Geometry: see drawing. Coordinates: mm, zero at the bounding-box minimum. A direction names the side the tool comes from. Coordinates: 2 decimals unless noted, no trailing zeros. Order: outer loops, then holes, each group sorted by start corner. A loop starts at its lowest first (then second) coordinate and runs counter-clockwise, first axis right, second up.
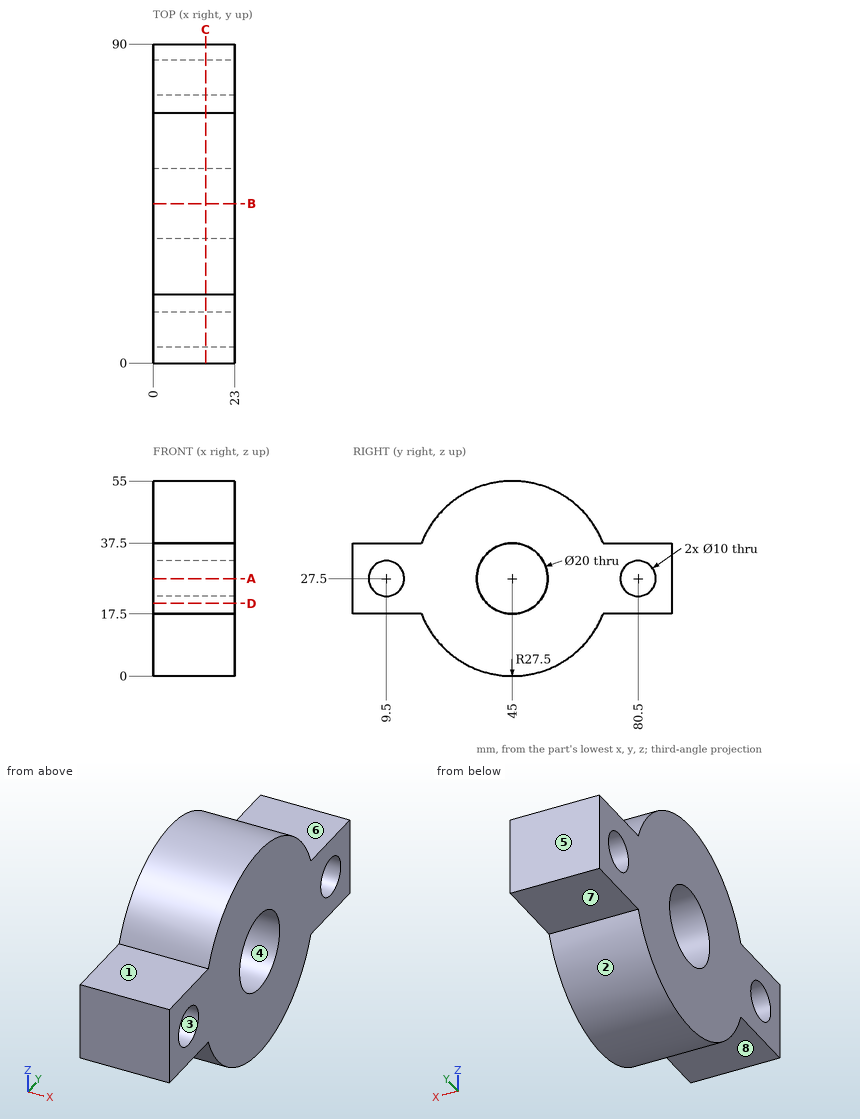
Q1. Section query B-B on y = 45. Output: boundary loops of the cut face in (x, z), plus the area to 3 significant figures.
Solutions:
outline: (0, 0) - (23, 0) - (23, 17.5) - (0, 17.5) - close; (0, 37.5) - (23, 37.5) - (23, 55) - (0, 55) - close
area: 805 mm2
Q2. Section query D-D on z = 20.5. Output: boundary loops of the cut face in (x, y), plus the area to 3 significant figures.
Solutions:
outline: (0, 0) - (23, 0) - (23, 37.86) - (0, 37.86) - close; (0, 52.14) - (23, 52.14) - (23, 90) - (0, 90) - close
area: 1,740 mm2
Q3. Material intervals for line 1 along Z through (x, y) = (11, 80.5); line 2 along Y through (x, z) = (17.5, 29); line 3 along Z through (x, y) = (3, 85), sorted ascending.
Solutions:
line 1: z = 17.5 to 22.5, 32.5 to 37.5
line 2: y = 0 to 4.73, 14.27 to 35.11, 54.89 to 75.73, 85.27 to 90
line 3: z = 17.5 to 25.32, 29.68 to 37.5
Q4. Pull-direction query (Z, two-part tool) for the marked faces 1, 2, 3 and 4; classes: pulls with the +Z half, pulls with the -Z half, needs draft (parallel to the pull), parting line crosses it, or undercut.
Solutions:
face 1: pulls with the +Z half
face 2: pulls with the -Z half
face 3: undercut
face 4: undercut
Q5. Set-up query: the marked faces 5, 6, 7 and 8. Return all of +Z, -Z, +X, -X, +Y, -Y with unobstructed straight access to the full face (end or side cutting, diameter ignored); none if empty.
Solutions:
face 5: +Z, -Z, +X, -X, +Y
face 6: +Z, +X, -X, +Y
face 7: -Z, +X, -X, +Y
face 8: -Z, +X, -X, -Y
Q6. Section query A-A on z = 27.5. Output: boundary loops of the cut face in (x, y), plus the area to 3 significant figures.
Solutions:
outline: (0, 0) - (23, 0) - (23, 4.5) - (0, 4.5) - close; (0, 14.5) - (23, 14.5) - (23, 35) - (0, 35) - close; (0, 55) - (23, 55) - (23, 75.5) - (0, 75.5) - close; (0, 85.5) - (23, 85.5) - (23, 90) - (0, 90) - close
area: 1,150 mm2
Q7. Section query C-C on x = 14.75. Output: boundary loops of the cut face in (y, z), plus the area to 3 significant figures.
Solutions:
outline: (0, 17.5) - (19.38, 17.5) arc R27.5 ccw to (70.62, 17.5) - (90, 17.5) - (90, 37.5) - (70.62, 37.5) arc R27.5 ccw to (19.38, 37.5) - (0, 37.5) - close; hole circle Ø10 at (9.5, 27.5); hole circle Ø20 at (45, 27.5); hole circle Ø10 at (80.5, 27.5)
area: 2,630 mm2
Q8. Pin query (flat end, axial travel): P1, Ø6, axis at x = 10.5, y = 83.5, coming from the +Z side; P2, Ø1, axis at x = 6, y = 76, coming from the -Z side; P3, Ø8, axis at x = 8, z = 9, coming from the -Y side. Return the tip coordinate at first contact, or that it passes through.
Solutions:
P1: stops at z = 37.5
P2: stops at z = 17.5
P3: stops at y = 21.63
